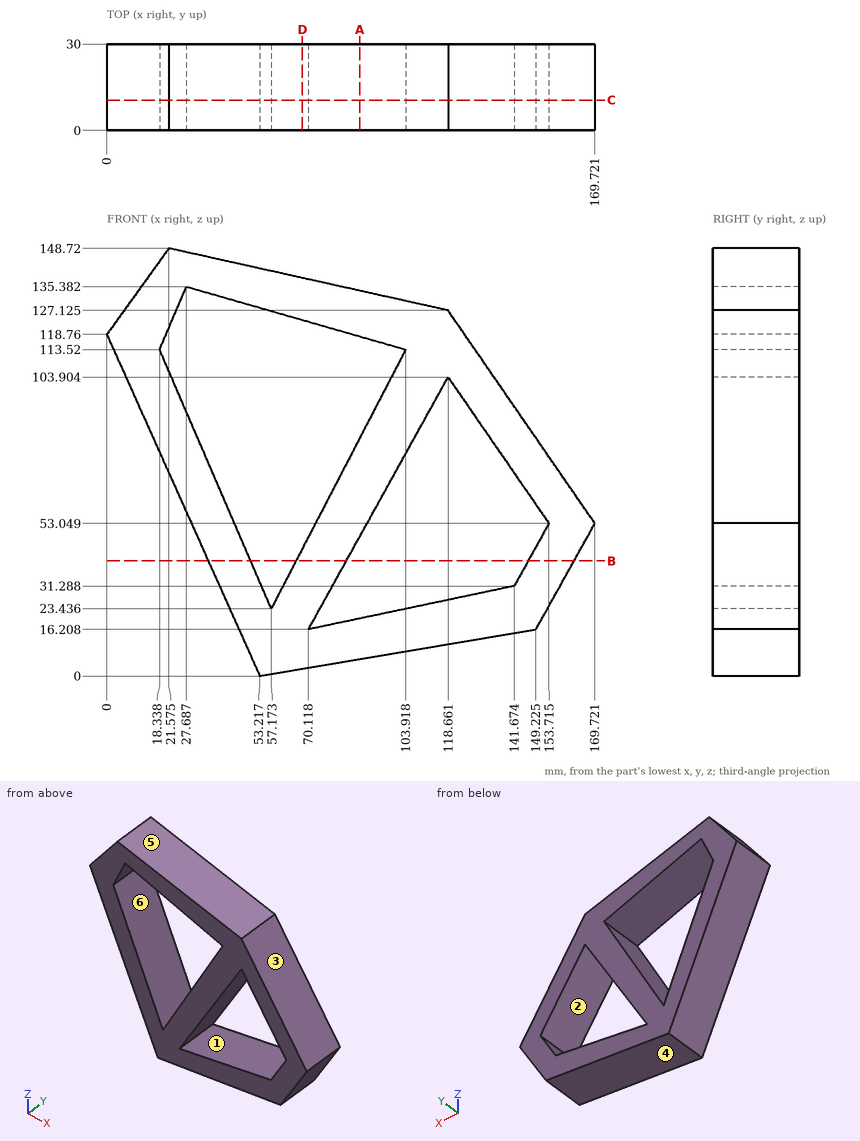
Geometry: see drawing. Coordinates: mm, zero at the bounding-box minimum. A direction names the side the tool comes from. Round coordinates to 2 decimals unless told otherwise and drop trailing zeros. Write each loop counter-clockwise with the first axis right and the second up, starting at its lowest first coordinate (ties: lowest second). Pieces come first, ordered by that corner, then holes. Notation, with made-up numbers: (15.25, 51.25) -> (56.25, 51.25) arc R17 ccw to (56.25, 81.25) -> close; hole circle Ø3 at (18.5, 52.25). An arc over 180 degrees is marked (long way). Answer as CSV lines item,"result".
1. Section B-B (z = 40). Return the cut outline in (x, y) (1 decimal), plus the area to 3 significant figures.
Geometry says:
outline,"(35.3, 0) -> (50, 0) -> (50, 30) -> (35.3, 30) -> close; (65.8, 0) -> (83.3, 0) -> (83.3, 30) -> (65.8, 30) -> close; (146.5, 0) -> (162.5, 0) -> (162.5, 30) -> (146.5, 30) -> close"
area,"1,450 mm^2"
2. Ray query, L1, parallel to Z at x = 86, y = 27.5 (1 decimal); L2, parallel to X at y = 27.75, z = 73 (1 decimal); L3, parallel to Z at x = 118.5, y = 10.75 (1 decimal). Return the intervals inside material, ascending. Write a range as [from, to].
Geometry says:
L1,"z = [5.5, 19.6], [44.9, 79], [118.7, 134.4]"
L2,"x = [20.5, 35.8], [82.9, 101.6], [140, 156]"
L3,"z = [11, 26.4], [103.6, 127.2]"
3. Section A-A (x = 88). Return the cut outline in (y, z) (1 decimal).
Geometry says:
outline,"(0, 5.9) -> (30, 5.9) -> (30, 20) -> (0, 20) -> close; (0, 48.5) -> (30, 48.5) -> (30, 82.8) -> (0, 82.8) -> close; (0, 118.1) -> (30, 118.1) -> (30, 133.9) -> (0, 133.9) -> close"
4. Mould query, pull axis Z, two halves, no side actions, for the marked faces 1, 2, 3 and 4. Classes: +Z half, -Z half, draft (parallel to the pull), parting line (faces both ways), or undercut.
Geometry says:
face 1,"undercut"
face 2,"undercut"
face 3,"+Z half"
face 4,"-Z half"
5. Reachability of the marked faces 5 and 6 from +Z, -Z, +X, -X, +Y, -Y: full face, straight path, thin tool, end or side. Return the list, or none.
Geometry says:
face 5,"+Z, +X, +Y, -Y"
face 6,"+Y, -Y"
6. Contact query for flat-ended pins moving along their axis: P1, Ø8, axis at y = 15.5, z = 37, coming from the +X side; P2, Ø5, axis at y = 25, z = 59, coming from the +X side; P3, Ø1.5, axis at x = 116, y = 3.5, coming from the -Z side; P4, Ø6, axis at x = 36, z = 60.5, coming from the -Y side. Output: stop coordinate, or through.
Geometry says:
P1,"stops at x = 163.02"
P2,"stops at x = 167.34"
P3,"stops at z = 10.47"
P4,"stops at y = 0"
7. Section D-D (x = 68). Return the cut outline in (y, z) (1 decimal), plus the area to 3 significant figures.
Geometry says:
outline,"(0, 2.5) -> (30, 2.5) -> (30, 44.3) -> (0, 44.3) -> close; (0, 123.8) -> (30, 123.8) -> (30, 138.4) -> (0, 138.4) -> close"
area,"1,690 mm^2"
8. Section C-C (y = 10.5). Return the cut outline in (x, z) (1 decimal), plus the area to 3 significant figures.
Geometry says:
outline,"(0, 118.8) -> (53.2, 0) -> (149.2, 16.2) -> (169.7, 53) -> (118.7, 127.1) -> (21.6, 148.7) -> close; hole (18.3, 113.5) -> (57.2, 23.4) -> (103.9, 113.5) -> (27.7, 135.4) -> close; hole (70.1, 16.2) -> (141.7, 31.3) -> (153.7, 53) -> (118.7, 103.9) -> close"
area,"7,980 mm^2"
